Can you work these out from the model? Positions are in its coordinate system, mm. A direction names the side the tool comes from. Give positions to 0.01 mm unless a question says otherwise; leave off trailing zeros. Write each loop counter-clockwise with the first axis right and the second up, starting at its lowest first coordinate (ties: lowest second). Pieces come first, ordered by that corner, then holes.
1. Suppose I cut it at C-C (y = 6.8). Please give me the cut outline in (x, z), and give its area (3 significant figures).
2. Suppose I cut it at A-A (y = -14.4). Please give me the cut outline in (x, z).
3. Suppose I cut it at B-B (z = 3.25). Please give me the cut outline in (x, y), and give its area (3 significant figures).
4. Thinking about a two-plate mould opening in Y: for faces 1 (the cylindrical face through (-5.713, -15.115, 0.225)), 2 (the flat face through (-6.65, -13, 0)), 3 (the cylindrical face through (-14.65, 9.02, -1.15)), 4 (the cylindrical face through (-5.713, 13.685, 0.225)), which applies, pulls with the +Y half, pulls with the -Y half, needs draft (parallel to the pull), parting line crosses it, or undercut?
5. If I drill on probe 1 along Z at (x, y) = (-5.2, 14.4); probe 2 along X at (y, z) = (-12, 2.5); probe 3 along X at (y, z) = (3, 3.5), over which ranges is the centre line in solid material (lowest first)?
6. Suppose I cut it at D-D (z = -2). Please give me the cut outline in (x, y).
7. On a 3-axis mill with a long thin cutter (end or side, diameter ignored), from which of +Z, -Z, +X, -X, +Y, -Y can I reach the whole of each face in a straight line? I mean faces 5 (the flat face through (-4.75, -13, 0)), 6 (the flat face through (-4.75, 13, 0)), 7 (the flat face through (-6.65, 13, 0)), 8 (the flat face through (-10, -11.5, 0)). Say none if no direction works.
8. I'm going to push flat-ended pins straight in: pin 1 (2.5 mm diameter, centred on y = -14.4, z = 0, fed in from -X); pin 2 (2 mm diameter, centred on x = -11.5, z = -2.5, fed in from +Y); pin 3 (2 mm diameter, centred on y = 3.5, z = 2.5, fed in from -X); pin 4 (1.4 mm diameter, centred on y = 14.4, z = 0, fed in from +X). Where does each tip first touch, or does it pass through?
```python
from build123d import *

# Parameters (mm, degrees)
BOSS_EXTRUDE1_DEPTH = 4.65
SKETCH3_W           = 3.05
SKETCH3_H           = 2.5
SKETCH4_R           = 0.75
CUT_EXTRUDE1_DEPTH  = 10


with BuildPart() as part:
    # Sketch1 → Boss-Extrude1 (new, symmetric)
    with BuildSketch(Plane.XY):
        Polygon((-4.75, 11.5), (-4.75, 16), (-6.65, 16), (-6.65, 11.5), (-13.15, 11.5), (-13.15, -11.5), (-6.65, -11.5), (-6.65, -16), (-4.75, -16), (-4.75, -11.5), (13.15, -11.5), (13.15, 11.5), align=None)
    extrude(amount=BOSS_EXTRUDE1_DEPTH, both=True)

    # Sketch3 → Revolve1 (revolve)
    with BuildSketch(Plane.XY, mode=Mode.PRIVATE) as revolve1_sk:
        with Locations((-14.675, 8.05)):
            Rectangle(SKETCH3_W, SKETCH3_H)
    revolve(revolve1_sk.sketch.rotate(Axis((-13.15, 6.8, 0), (-1, 0, 0)), 90), axis=Axis((-13.15, 6.8, 0), (-1, 0, 0)))

    # Sketch4 → Cut-Extrude1 (cut)
    with BuildSketch(Plane.ZY.offset(6.65)):
        with Locations(Location((0, 14.4, 0), (0, 0, 270))):
            Circle(SKETCH4_R)
        with Locations(Location((0, -14.4, 0), (0, 0, 270))):
            Circle(SKETCH4_R)
    extrude(amount=-CUT_EXTRUDE1_DEPTH, mode=Mode.SUBTRACT)


solid = part.part
```
Checks:
1. outline: (-16.2, -2.5) - (-13.15, -2.5) - (-13.15, -4.65) - (13.15, -4.65) - (13.15, 4.65) - (-13.15, 4.65) - (-13.15, 2.5) - (-16.2, 2.5) - close
1. area: 260 mm2
2. outline: (-6.65, -4.65) - (-4.75, -4.65) - (-4.75, -0.75) - (-6.65, -0.75) - close; (-6.65, 0.75) - (-4.75, 0.75) - (-4.75, 4.65) - (-6.65, 4.65) - close
3. outline: (-13.15, -11.5) - (-6.65, -11.5) - (-6.65, -16) - (-4.75, -16) - (-4.75, -11.5) - (13.15, -11.5) - (13.15, 11.5) - (-4.75, 11.5) - (-4.75, 16) - (-6.65, 16) - (-6.65, 11.5) - (-13.15, 11.5) - close
3. area: 622 mm2
4. face 1: undercut
4. face 2: needs draft
4. face 3: parting line crosses it
4. face 4: undercut
5. probe 1: z = -4.65 to -0.75, 0.75 to 4.65
5. probe 2: x = -6.65 to -4.75
5. probe 3: x = -13.15 to 13.15
6. outline: (-16.2, 5.3) - (-13.15, 5.3) - (-13.15, -11.5) - (-6.65, -11.5) - (-6.65, -16) - (-4.75, -16) - (-4.75, -11.5) - (13.15, -11.5) - (13.15, 11.5) - (-4.75, 11.5) - (-4.75, 16) - (-6.65, 16) - (-6.65, 11.5) - (-13.15, 11.5) - (-13.15, 8.3) - (-16.2, 8.3) - close
7. face 5: +Z, -Z, +X, -Y
7. face 6: +Z, -Z, +X, +Y
7. face 7: +Z, -Z, -X, +Y
7. face 8: +Z, -Z, -X, -Y
8. pin 1: stops at x = -6.65
8. pin 2: stops at y = 11.5
8. pin 3: stops at x = -13.15
8. pin 4: passes through
